CAD build for the part. Positions are in the model's coordinates, mm. Face numbers are marked on the shaded views. A direction names the side the tool comes from. Coordinates: 2 decimals unless noted, no trailing zeros. Order: outer loops, then holes, each group sorted by start corner. A loop starts at its lowest first (then second) coordinate and runs counter-clockwise, first axis right, second up.
from build123d import *

# Parameters (mm, degrees)
F2_DEPTH = 37.846
F1_W     = 73.8076716661
F1_H     = 49.2051169276
F3_DEPTH = 38.1
F4_T     = 9.0678


with BuildPart() as f2:
    # F0 (on Top) → F2 (new body, symmetric)
    with BuildSketch(Plane.XY):
        Polygon((50.624661522, -33.5625614026), (50.624661522, 33.5625614026), (0, 11.3709298894), (0, -11.5776741877), align=None)
        Polygon((0, 11.3709298894), (-50.624661522, 33.5625614026), (-50.624661522, -33.5625614026), (0, -11.5776741877), align=None)
        Polygon((0, 11.3709298894), (50.624661522, 33.5625614026), (-50.624661522, 33.5625614026), align=None)
        Polygon((-50.624661522, -33.5625614026), (50.624661522, -33.5625614026), (0, -11.5776741877), align=None)
    extrude(amount=F2_DEPTH, both=True)

    # F1 (on Front) → F3 (join)
    with BuildSketch(Plane.XZ):
        Rectangle(F1_W, F1_H)
    extrude(amount=F3_DEPTH)

    # F4
    f4_openings = [f2.faces().sort_by_distance(p)[0] for p in [
        (0, 33.562561, 0),
    ]]
    offset(amount=F4_T, openings=f4_openings, kind=Kind.INTERSECTION)


solid = f2.part
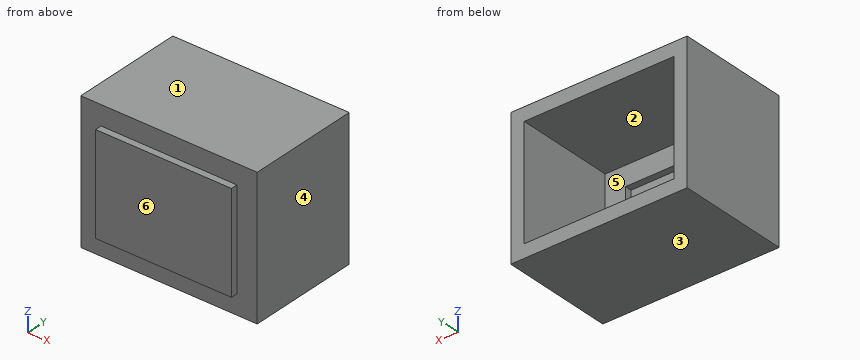
1) Slice it at B-B (z = -16). List the corners of the cut face in (x, y), plus the area to 3 significant figures.
2) Drill centre lines: probe 1 along Z at (x, y) = (-49, -12); probe 2 along X at (y, z) = (-31, -21); probe 3 along Z at (x, y) = (-8.5, -36). Where is each one in solid material? Low to high.
3) Two-plate mould, pull along Z, no slides. Class the marked faces 1, 2, 3 and 4: released by +Z, released by -Z, zero draft, split by the parting line, or undercut.
4) Pin check, flat tips, straight feed: P1, Ø2.5, axis at x = -13, y = -46, coming from the -Z side; P2, Ø2.5, axis at y = -44.5, z = 0.5, coming from the -X side; P3, Ø2.5, axis at y = -45, z = -12.5, coming from the +X side. Stop position of each tip, or through.
5) Slice it at A-A (x = 49). List the corners of the cut face in (y, z).
6) Slice it at C-C (y = 10.5). List the corners of the cut face in (x, z), plus the area to 3 significant figures.
7) Slice it at D-D (x = 3.5). List the corners of the cut face in (y, z).
8) Which spindle directions (+Z, -Z, +X, -X, +Y, -Y) get a long thin tool onto all of the face, cutting with end or side? Do the marked faces 5 and 6. Say none if no direction does.
Worked out:
1. outline: (-59.69, -42.63) - (-45.97, -42.63) - (-45.97, -47.17) - (45.97, -47.17) - (45.97, -42.63) - (59.69, -42.63) - (59.69, 33.56) - (50.62, 33.56) - (50.62, -33.56) - (36.9, -33.56) - (36.9, -38.1) - (-36.9, -38.1) - (-36.9, -33.56) - (-50.62, -33.56) - (-50.62, 33.56) - (-59.69, 33.56) - close
1. area: 2,380 mm2
2. probe 1: z = -46.91 to -37.85, 37.85 to 46.91
2. probe 2: x = -59.69 to -50.62, 50.62 to 59.69
2. probe 3: z = -46.91 to -24.6, 24.6 to 46.91
3. face 1: released by +Z
3. face 2: undercut
3. face 3: released by -Z
3. face 4: zero draft
4. P1: stops at z = -33.67
4. P2: stops at x = -45.97
4. P3: stops at x = 45.97
5. outline: (-42.63, -46.91) - (33.56, -46.91) - (33.56, -37.85) - (-33.56, -37.85) - (-33.56, 37.85) - (33.56, 37.85) - (33.56, 46.91) - (-42.63, 46.91) - close
6. outline: (-59.69, -46.91) - (59.69, -46.91) - (59.69, 46.91) - (-59.69, 46.91) - close; hole (-50.62, -37.85) - (50.62, -37.85) - (50.62, 37.85) - (-50.62, 37.85) - close
6. area: 3,540 mm2
7. outline: (-47.17, -33.67) - (-42.63, -33.67) - (-42.63, -46.91) - (33.56, -46.91) - (33.56, -37.85) - (-33.56, -37.85) - (-33.56, -24.6) - (-38.1, -24.6) - (-38.1, 24.6) - (-33.56, 24.6) - (-33.56, 37.85) - (33.56, 37.85) - (33.56, 46.91) - (-42.63, 46.91) - (-42.63, 33.67) - (-47.17, 33.67) - close
8. face 5: +Y
8. face 6: +Z, -Z, +X, -X, -Y
